Can you work these out from the drawing? Everything is in mm from the part's minimum corner. A direction names the side the tool comes from. Coordinates: 2 decimals unless noted, no trailing zeros. Order: outer loops, then holes, each group sorted by start corner. A loop starts at its lowest first (then second) coordinate and runs counter-clockwise, first axis right, second up. Notation, with made-up numbers: (16, 6) -> (28, 6) arc R7 cw to (28, 14) -> close; hole circle Ø8 at (73.25, 3). An arc over 180 degrees is marked (long way). Put each result on its own line as item: value. Start each with the question number.
Q1. Will these pins go through, and if not, where does the flat tip stop? pin 1 (3.5 mm diameter, centred on x = 4.5, z = 10.5, fed in from -Y); pin 2 (3 mm diameter, centred on y = 14.5, z = 15, fed in from +X); pin 3 (2 mm diameter, centred on x = 50, z = 11, fed in from +Y).
Q2. If we section it at C-C (z = 1.75): Please give me the cut outline in (x, y), and give its area (3 significant figures).
Q3. If we section it at B-B (x = 37.35): Please give me the cut outline in (y, z), and give its area (4 significant figures).
Q4. For the marked faces 1, 2, 3 and 4, which set-ups out of +Z, -Z, +X, -X, +Y, -Y let a thin tool reach every point of the face, with its end or its side?
Q5. Please list where these lines run through material, in increasing order: line 1 along Z through (x, y) = (52, 29.1); line 2 along X through (y, z) = (7, 5.5); line 3 along X through (y, z) = (28.45, 15).
Q6. If we section it at D-D (z = 10): Please give me the cut outline in (x, y).
Q7. If we section it at A-A (x = 52): Please give me the cut outline in (y, z).
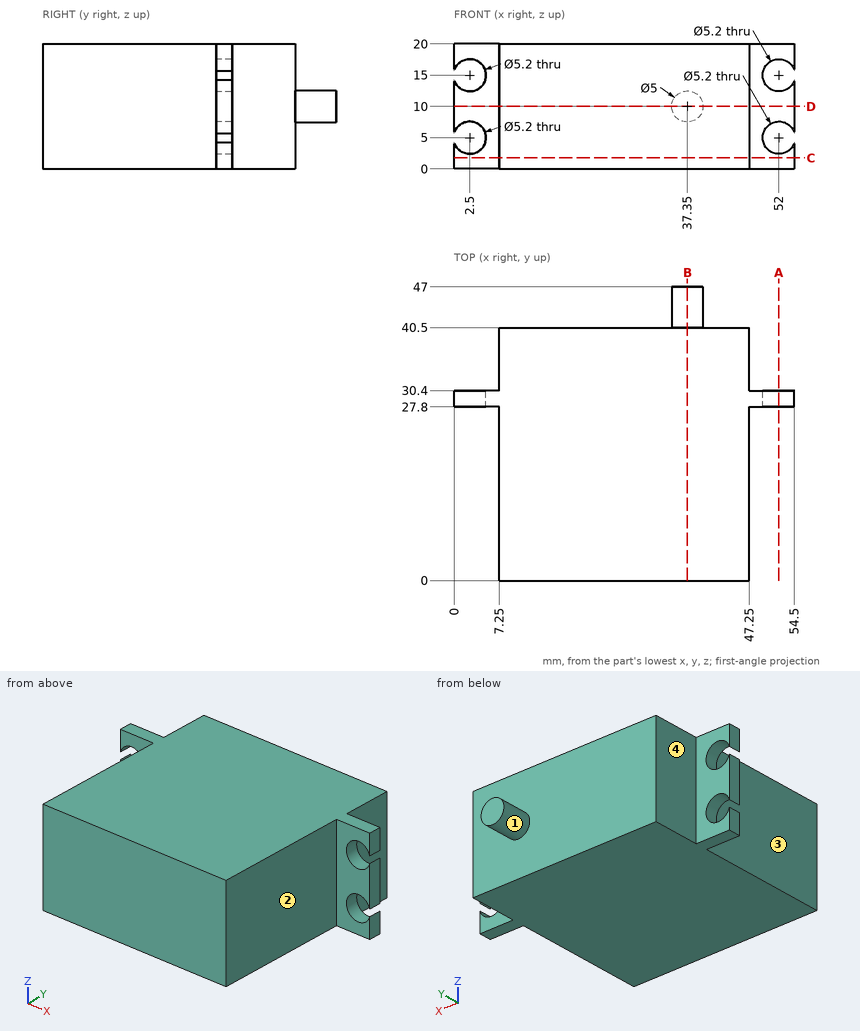
The answers:
1. pin 1: y = 27.8
1. pin 2: x = 47.25
1. pin 3: y = 30.4
2. outline: (0, 27.8) -> (7.25, 27.8) -> (7.25, 0) -> (47.25, 0) -> (47.25, 27.8) -> (54.5, 27.8) -> (54.5, 30.4) -> (47.25, 30.4) -> (47.25, 40.5) -> (7.25, 40.5) -> (7.25, 30.4) -> (0, 30.4) -> close
2. area: 1,660 mm^2
3. outline: (0, 0) -> (40.5, 0) -> (40.5, 7.5) -> (47, 7.5) -> (47, 12.5) -> (40.5, 12.5) -> (40.5, 20) -> (0, 20) -> close
3. area: 842.5 mm^2
4. face 1: +Y
4. face 2: +Z, -Z, +X, -Y
4. face 3: +Z, -Z, -X, -Y
4. face 4: +Z, -Z, -X, +Y
5. line 1: 0 to 2.4, 7.6 to 12.4, 17.6 to 20
5. line 2: 7.25 to 47.25
5. line 3: 5.1 to 49.4
6. outline: (0, 27.8) -> (7.25, 27.8) -> (7.25, 0) -> (47.25, 0) -> (47.25, 27.8) -> (54.5, 27.8) -> (54.5, 30.4) -> (47.25, 30.4) -> (47.25, 40.5) -> (39.85, 40.5) -> (39.85, 47) -> (34.85, 47) -> (34.85, 40.5) -> (7.25, 40.5) -> (7.25, 30.4) -> (0, 30.4) -> close
7. outline: (27.8, 0) -> (30.4, 0) -> (30.4, 2.4) -> (27.8, 2.4) -> close; (27.8, 7.6) -> (30.4, 7.6) -> (30.4, 12.4) -> (27.8, 12.4) -> close; (27.8, 17.6) -> (30.4, 17.6) -> (30.4, 20) -> (27.8, 20) -> close
